For this review, take the finished solid that the model builds, in its own axes (mm). A direction names the side the tool comes from. Coordinates: 2 decimals unless noted, no trailing zeros. Write each loop counter-clockwise with the first axis right and the second up, starting at its lowest first coordinate (ties: lowest second). Pieces come first, ordered by that corner, then holes. Notation, with made-up numbers: (52.25, -8) -> (81.25, -8) arc R24 cw to (81.25, 23) -> close; hole circle Ø8 at (1, -2). An arc over 180 degrees is marked (long way). Put each result on its own line as item: value. Start each with the question number.
Item 1: For faces 4 (the flat face through (76.2, -8, 40)), 5 (the flat face through (88.9, -28, 8)), 6 (the flat face through (52, -25.4, 8)), 7 (the flat face through (12.7, -28, 8)), 8 (the cylindrical face through (98.698, -7.727, 60.748)), list the 3-axis set-ups (+Z, -Z, +X, -X, +Y, -Y) from which the entire face can be reached by the end or side of a thin tool; tool diameter is ignored.
Item 2: To check wall thickness, follow L1, parallel to X at y = -6.25, z = 50.8; L2, parallel to Z at x = 12, y = -3; L3, parallel to X at y = -5, z = 40.5. State the ranges of each line that lie inside material, in increasing order.
Item 3: Consider section D-D on z = 50.8. Give the boundary of the cut face in (x, y).
Item 4: Insertion check: P1, Ø5, axis at x = 74, z = 30, coming from the +Y side; P2, Ø1.8, axis at y = -29, z = 11, coming from the +X side; P3, Ø5, axis at y = -29, z = 4, coming from the -X side; P4, Ø10.5, axis at x = 81, z = 35.5, coming from the -Y side. Each pin has a flat end and moves straight along its axis. Give the tip position at first contact, or say it passes through.
Item 5: The part is to be moulded in two halves that separate along X. For faces 1 (the flat face through (101.6, -8, 27)), 2 (the cylindrical face through (17.72, -7.51, 58.68)), 3 (the cylindrical face through (15.602, -37.888, 8.113)), say which applies: +X half, -X half, draft (parallel to the pull), parting line (faces both ways), or undercut.
Item 6: Consider section A-A on x = 51.5. Give the boundary of the cut face in (y, z), and give its area (3 significant figures).
Item 7: Consider section B-B on z = 33. Give the boundary of the cut face in (x, y).
Item 8: Consider section C-C on y = -13.5. Give the boundary of the cut face in (x, z).
```python
from build123d import *

# Parameters (mm, degrees)
F2_DEPTH  = 40.64
F1_R      = 9.3438702408
F3_DEPTH  = 40.641
F5_START  = 16.002
F4_W      = 101.6
F4_H      = 25.4
F5_DEPTH  = 47.499
F6_W      = 12.7
F6_H      = 16.002
F7_DEPTH  = 25.4
F8_R      = 9.652
F9_R      = 9.652
F11_DEPTH = 16.003
F12_R     = 9.652


with BuildPart() as f2:
    # F0 (on Front) → F2 (new body)
    with BuildSketch(Plane.XZ):
        Polygon((0, 63.5), (0, 0), (101.6, 0), (101.6, 63.5), (76.2, 63.5), (76.2, 16.002), (25.4, 16.002), (25.4, 63.5), align=None)
    extrude(amount=F2_DEPTH)

    # F1 (on face) → F3 (cut, through all)
    with BuildSketch(Plane.XZ):
        with Locations((12.7, 50.8)):
            Circle(F1_R)
        with Locations((88.9, 50.8)):
            Circle(F1_R)
    extrude(amount=F3_DEPTH, mode=Mode.SUBTRACT)

    # F4 (on Top) → F5 (cut)
    with BuildSketch(Plane.XY.offset(F5_START)):
        with Locations((50.8, -27.94)):
            Rectangle(F4_W, F4_H)
    extrude(amount=F5_DEPTH, mode=Mode.SUBTRACT)

    # F6 (on face) → F7 (cut)
    with BuildSketch(Plane.XZ.offset(40.64)):
        with Locations((6.35, 8.001)):
            Rectangle(F6_W, F6_H)
        with Locations((95.25, 8.001)):
            Rectangle(F6_W, F6_H)
    extrude(amount=-F7_DEPTH, mode=Mode.SUBTRACT)

    # F8
    f8_edges = [f2.edges().sort_by_distance(p)[0] for p in [
        (25.4, -7.62, 63.5),
        (0, -7.62, 63.5),
        (76.2, -7.62, 63.5),
        (101.6, -7.62, 63.5),
    ]]
    fillet(f8_edges, radius=F8_R)

    # F9
    f9_edges = [f2.edges().sort_by_distance(p)[0] for p in [
        (12.7, -40.64, 8.001),
        (88.9, -40.64, 8.001),
        (12.7, -15.24, 8.001),
        (88.9, -15.24, 8.001),
    ]]
    fillet(f9_edges, radius=F9_R)

    # F10 (on face) → F11 (cut, through all)
    with BuildSketch(Plane.XY.offset(16.002)):
        with BuildLine():
            ThreePointArc((22.7949339896, -25.4), (16.4449339896, -31.75), (22.7949339896, -38.1))
            Line((22.7949339896, -38.1), (79.5431733131, -38.1))
            ThreePointArc((79.5431733131, -38.1), (85.8931733131, -31.75), (79.5431733131, -25.4))
            Line((79.5431733131, -25.4), (22.7949339896, -25.4))
        make_face()
    extrude(amount=-F11_DEPTH, mode=Mode.SUBTRACT)

    # F12
    f12_edges = [f2.edges().sort_by_distance(p)[0] for p in [
        (25.4, -7.62, 16.002),
        (76.2, -7.62, 16.002),
    ]]
    fillet(f12_edges, radius=F12_R)


solid = f2.part
```
Return value:
1. face 4: +Z, +Y, -Y
1. face 5: +Z, -Z, +X, -Y
1. face 6: +Z, -Z
1. face 7: +Z, -Z, -X, -Y
1. face 8: +Z, +X, +Y, -Y
2. L1: 0 to 3.36, 22.04 to 25.4, 76.2 to 79.56, 98.24 to 101.6
2. L2: 0 to 41.48, 60.12 to 63.5
2. L3: 0 to 25.4, 76.2 to 101.6
3. outline: (0, -15.24) -> (3.36, -15.24) -> (3.36, 0) -> (0, 0) -> close; (22.04, -15.24) -> (25.4, -15.24) -> (25.4, 0) -> (22.04, 0) -> close; (76.2, -15.24) -> (79.56, -15.24) -> (79.56, 0) -> (76.2, 0) -> close; (98.24, -15.24) -> (101.6, -15.24) -> (101.6, 0) -> (98.24, 0) -> close
4. P1: y = 0
4. P2: x = 88.9
4. P3: x = 12.7
4. P4: y = -15.24
5. face 1: +X half
5. face 2: undercut
5. face 3: -X half
6. outline: (-40.64, 0) -> (-38.1, 0) -> (-38.1, 16) -> (-40.64, 16) -> close; (-25.4, 0) -> (0, 0) -> (0, 16) -> (-25.4, 16) -> close
6. area: 447 mm^2
7. outline: (0, -15.24) -> (25.4, -15.24) -> (25.4, 0) -> (0, 0) -> close; (76.2, -15.24) -> (101.6, -15.24) -> (101.6, 0) -> (76.2, 0) -> close
8. outline: (0, 0) -> (101.6, 0) -> (101.6, 53.85) arc R9.65 ccw to (91.95, 63.5) -> (85.85, 63.5) arc R9.65 ccw to (76.2, 53.85) -> (76.2, 25.65) arc R9.65 cw to (66.55, 16) -> (35.05, 16) arc R9.65 cw to (25.4, 25.65) -> (25.4, 53.85) arc R9.65 ccw to (15.75, 63.5) -> (9.65, 63.5) arc R9.65 ccw to (0, 53.85) -> close; hole circle Ø18.69 at (12.7, 50.8); hole circle Ø18.69 at (88.9, 50.8)
